Here's how the part is built. I have some questions about the finished solid (model axes, mm). A direction names the side the tool comes from. Give positions to 0.01 mm unless a question says otherwise; leave off trailing zeros. Write each loop counter-clockwise with the first axis right and the second up, starting at its lowest first coordinate (ties: lowest second). Pieces come first, ordered by that corner, then holes. Notation, with made-up numbers: (-16, 57.5) - (24, 57.5) arc R14 cw to (24, 64.5) - close; hole circle Ø2 at (18.5, 18). An arc over 180 degrees is marked (long way). Write each question's results on one line, items separated by ' | '. Start each with the question number.
Item 1: Suppose I cut it at C-C on y = 12. List the corners of the cut face in (x, z) for me.
Item 2: Suppose I cut it at D-D on x = 23.5. List the corners of the cut face in (y, z) for me.
Item 3: Suppose I cut it at B-B on z = -29.5. List the corners of the cut face in (x, y) for me.
Item 4: Please list where these lines run through material, in increasing order: line 1 along Y through (x, z) = (3, -37.7); line 2 along X through (y, z) = (14.5, -36); line 3 along Z through (x, y) = (-8, 11).
Item 5: We'd pull the mould along Y, two halves only. Please class faces 4 (the flat face through (-2, 13, -20)), 5 (the flat face through (3, 16, -30)), 6 (the cylindrical face through (-9.703, -1.014, -38.521)): +Y half, -Y half, draft (parallel to the pull), parting line (faces both ways), or undercut.
Item 6: Which directions (+Z, -Z, +X, -X, +Y, -Y) give clear straight access to the entire face, cutting with the end or side of a thin tool? Please do faces 1 (the flat face through (7, 12, -30)), 2 (the flat face through (3, 5, -29)), 3 (the flat face through (10, 12, -29)).
Item 7: Will these pins go through, and if not, where does the flat tip stop? P1, Ø6.5, axis at y = 14, z = -30, coming from the +X side; P2, Ø6.5, axis at x = 1.5, z = -26, coming from the -Y side; P3, Ø4, axis at x = -13, z = -33.5, coming from the +Y side; P4, Ø5, axis at x = -5, y = -7, coming from the +Z side.
Item 8: Suppose I cut it at A-A on x = 3. List the corners of the cut face in (y, z) for me, then the cut area to 3 significant figures.
```python
from build123d import *

# Parameters (mm, degrees)
CYLINDER018_R     = 2
CYLINDER018_DEPTH = 3
CYLINDER019_R     = 2
CYLINDER019_DEPTH = 3
CYLINDER014_R     = 20
CYLINDER014_DEPTH = 3
CYLINDER021_R     = 2
CYLINDER021_DEPTH = 3
CYLINDER017_R     = 20
CYLINDER017_DEPTH = 3
CYLINDER016_R     = 20
CYLINDER016_DEPTH = 3
CYLINDER015_R     = 20
CYLINDER015_DEPTH = 3
CYLINDER020_R     = 2
CYLINDER020_DEPTH = 3
BOX016_W          = 8
BOX016_H          = 8
BOX016_DEPTH      = 20
BOX018_W          = 54
BOX018_H          = 54
BOX018_DEPTH      = 3
BOX015_W          = 14
BOX015_H          = 15
BOX015_DEPTH      = 20


with BuildPart() as zylinder018:
    # Cylinder018 → Cylinder018 (new body)
    with BuildSketch(Plane(origin=(3, -9, -40), x_dir=(1, 0, 0), z_dir=(0, 0, 1))):
        Circle(CYLINDER018_R)
    extrude(amount=CYLINDER018_DEPTH)


with BuildPart() as zylinder019:
    # Cylinder019 → Cylinder019 (new body)
    with BuildSketch(Plane(origin=(3, 33, -40), x_dir=(1, 0, 0), z_dir=(0, 0, 1))):
        Circle(CYLINDER019_R)
    extrude(amount=CYLINDER019_DEPTH)


with BuildPart() as zylinder014:
    # Cylinder014 → Cylinder014 (new body)
    with BuildSketch(Plane(origin=(30, -15, -40), x_dir=(1, 0, 0), z_dir=(0, 0, 1))):
        Circle(CYLINDER014_R)
    extrude(amount=CYLINDER014_DEPTH)


with BuildPart() as zylinder021:
    # Cylinder021 → Cylinder021 (new body)
    with BuildSketch(Plane(origin=(-18, 12, -40), x_dir=(1, 0, 0), z_dir=(0, 0, 1))):
        Circle(CYLINDER021_R)
    extrude(amount=CYLINDER021_DEPTH)


with BuildPart() as zylinder017:
    # Cylinder017 → Cylinder017 (new body)
    with BuildSketch(Plane(origin=(30, 39, -40), x_dir=(1, 0, 0), z_dir=(0, 0, 1))):
        Circle(CYLINDER017_R)
    extrude(amount=CYLINDER017_DEPTH)


with BuildPart() as zylinder016:
    # Cylinder016 → Cylinder016 (new body)
    with BuildSketch(Plane(origin=(-24, 39, -40), x_dir=(1, 0, 0), z_dir=(0, 0, 1))):
        Circle(CYLINDER016_R)
    extrude(amount=CYLINDER016_DEPTH)


with BuildPart() as zylinder015:
    # Cylinder015 → Cylinder015 (new body)
    with BuildSketch(Plane(origin=(-24, -15, -40), x_dir=(1, 0, 0), z_dir=(0, 0, 1))):
        Circle(CYLINDER015_R)
    extrude(amount=CYLINDER015_DEPTH)


with BuildPart() as zylinder020:
    # Cylinder020 → Cylinder020 (new body)
    with BuildSketch(Plane(origin=(24, 12, -40), x_dir=(1, 0, 0), z_dir=(0, 0, 1))):
        Circle(CYLINDER020_R)
    extrude(amount=CYLINDER020_DEPTH)


with BuildPart() as fusion009:
    # Box016 → Box016 (new body)
    with BuildSketch(Plane(origin=(-1, 8, -40), x_dir=(1, 0, 0), z_dir=(0, 0, 1))):
        with Locations((4, 4)):
            Rectangle(BOX016_W, BOX016_H)
    extrude(amount=BOX016_DEPTH)

    # Fusion009: union Zylinder018, Zylinder019, Zylinder014, Zylinder021, Zylinder017, Zylinder016, Zylinder015, Zylinder020
    add(zylinder018.part)
    add(zylinder019.part)
    add(zylinder014.part)
    add(zylinder021.part)
    add(zylinder017.part)
    add(zylinder016.part)
    add(zylinder015.part)
    add(zylinder020.part)


with BuildPart() as cube018:
    # Box018 → Box018 (new body)
    with BuildSketch(Plane(origin=(-24, -15, -40), x_dir=(1, 0, 0), z_dir=(0, 0, 1))):
        with Locations((27, 27)):
            Rectangle(BOX018_W, BOX018_H)
    extrude(amount=BOX018_DEPTH)


with BuildPart() as sockel:
    # Box015 → Box015 (new body)
    with BuildSketch(Plane(origin=(-4, 5, -40), x_dir=(1, 0, 0), z_dir=(0, 0, 1))):
        with Locations((7, 7.5)):
            Rectangle(BOX015_W, BOX015_H)
    extrude(amount=BOX015_DEPTH)

    # Fusion008: union Cube018
    add(cube018.part)

    # Cut004: cut Fusion009
    add(fusion009.part, mode=Mode.SUBTRACT)


solid = sockel.part
```
Checked values:
1) outline: (-24, -40) - (-20, -40) - (-20, -37) - (-24, -37) - close; (-16, -40) - (-1, -40) - (-1, -20) - (-4, -20) - (-4, -37) - (-16, -37) - close; (7, -40) - (22, -40) - (22, -37) - (10, -37) - (10, -20) - (7, -20) - close; (26, -40) - (30, -40) - (30, -37) - (26, -37) - close
2) outline: (3.91, -40) - (10.06, -40) - (10.06, -37) - (3.91, -37) - close; (13.94, -40) - (20.09, -40) - (20.09, -37) - (13.94, -37) - close
3) outline: (-4, 5) - (10, 5) - (10, 20) - (-4, 20) - close; hole (-1, 8) - (7, 8) - (7, 16) - (-1, 16) - close
4) line 1: y = -15 to -11, -7 to 8, 16 to 31, 35 to 39 | line 2: x = -4 to -1, 7 to 10 | line 3: z = -40 to -37
5) face 4: draft | face 5: undercut | face 6: -Y half
6) face 1: +Z, -Z | face 2: +Z, +X, -X, -Y | face 3: +Z, +X, +Y, -Y
7) P1: stops at x = 10 | P2: stops at y = 5 | P3: passes through | P4: stops at z = -37
8) outline: (-15, -40) - (-11, -40) - (-11, -37) - (-15, -37) - close; (-7, -40) - (8, -40) - (8, -20) - (5, -20) - (5, -37) - (-7, -37) - close; (16, -40) - (31, -40) - (31, -37) - (20, -37) - (20, -20) - (16, -20) - close; (35, -40) - (39, -40) - (39, -37) - (35, -37) - close | area: 233 mm^2
